Design review of the part built by this model. Coordinates are the model's own, in mm. A direction names the side the tool comes from. Give positions to 0.01 mm unless a question says otherwise; leave off trailing zeros. Loops run counter-clockwise (first coordinate to the right, second up) from the corner with the lowest first, then second, coordinate; pieces in that order, holes last. Notation, with made-up numbers: (30.5, -23.5) - (37.5, -23.5) arc R25 ccw to (37.5, 4.5) - close; hole circle Ø9 at (-39, 49). An arc over 180 degrees is marked (long way). Write each question's results on one line, items separated by ' | '.
from build123d import *

# Parameters (mm, degrees)
SKETCH1_R           = 3
BOSS_EXTRUDE1_DEPTH = 3.175


with BuildPart() as part:
    # Sketch1 → Boss-Extrude1 (new body)
    with BuildSketch(Plane.XY):
        with BuildLine():
            Line((25, 170), (175, 170))
            ThreePointArc((175, 170), (223.684930832, 189.383563894), (275, 200))
            Line((275, 200), (278.48892965, 170.203567833))
            ThreePointArc((278.48892965, 170.203567833), (228.984362684, 159.629140364), (182.323699215, 140))
            Line((182.323699215, 140), (17.676300785, 140))
            ThreePointArc((17.676300785, 140), (-27.163176857, 159.050053662), (-74.696057289, 169.732215313))
            add(Edge.make_bspline(
                [(-459.597813184, -125.74437106), (-458.167847661, -124.888859924), (-455.300989911, -123.160410804), (-449.693031194, -119.725805066), (-442.844497858, -115.430194443), (-434.897527213, -110.280573748), (-424.643042919, -103.410605598), (-412.446207366, -94.807407336), (-398.73286692, -84.425459971), (-385.875530014, -73.956655832), (-369.787206696, -59.850046206), (-355.152571956, -45.476802835), (-341.718077927, -30.784744771), (-332.160906415, -19.581186548), (-323.101555816, -8.241034683), (-311.630816912, 6.863649777), (-298.117522758, 25.605990916), (-282.395742384, 47.431562205), (-266.384320483, 68.25099024), (-249.34123977, 87.803395961), (-230.504956306, 105.928130356), (-212.601243201, 119.774018212), (-196.457396921, 130.048920131), (-183.303935629, 137.33205425), (-168.969219752, 144.162376514), (-153.317967868, 150.50005901), (-136.218766867, 156.296597686), (-120.658812709, 160.629761276), (-107.364076993, 163.767973943), (-96.958515184, 165.949209965), (-87.903435435, 167.618170459), (-80.445251901, 168.856738216), (-76.604810273, 169.448930821), (-74.696057289, 169.732215313)],
                knots=[0, 0, 0, 0, 0.007772041, 0.015544083, 0.031088165, 0.046632248, 0.06217633, 0.093264496, 0.124352661, 0.155440826, 0.186528991, 0.248705321, 0.279793487, 0.310881652, 0.341969817, 0.373057982, 0.435234312, 0.497410643, 0.559586973, 0.621763303, 0.683939634, 0.746115964, 0.777204129, 0.808292294, 0.83938046, 0.870468625, 0.90155679, 0.932644955, 0.948189038, 0.96373312, 0.979277203, 0.987049244, 0.994821285, 0.994821285, 0.994821285, 0.994821285], degree=3))
            Line((-459.597813184, -125.74437106), (-518.031074044, -125.74437106))
            Line((-518.031074044, -125.74437106), (-475, -100))
            add(Edge.make_bspline(
                [(-475, -100), (-419.540575809, -66.820070684), (-306.013905785, 34.036801702), (-257.635554762, 174.287094016), (-75, 200)],
                knots=[0, 0, 0, 0, 0.312223899, 1, 1, 1, 1], degree=3))
            ThreePointArc((-75, 200), (-23.684930832, 189.383563894), (25, 170))
        make_face()
        with Locations((-412.174499428, -75.74437106)):
            Circle(SKETCH1_R, mode=Mode.SUBTRACT)
        with Locations((-317.601811803, 24.25562894)):
            Circle(SKETCH1_R, mode=Mode.SUBTRACT)
        with Locations((-231.096695012, 124.25562894)):
            Circle(SKETCH1_R, mode=Mode.SUBTRACT)
        with Locations((-127.411512689, 174.25562894)):
            Circle(SKETCH1_R, mode=Mode.SUBTRACT)
        with Locations((100, 155)):
            Circle(SKETCH1_R, mode=Mode.SUBTRACT)
        with Locations((226.311251147, 174.505328628)):
            Circle(SKETCH1_R, mode=Mode.SUBTRACT)
        with Locations((-25.392583218, 174.221837866)):
            Circle(SKETCH1_R, mode=Mode.SUBTRACT)
    extrude(amount=BOSS_EXTRUDE1_DEPTH)


solid = part.part
(1) Take a section at B-B on z = 1.8. Count the separate pieces of the cut face and the enclosed holes in it, plus the area to 3 significant figures.
Answers below:
separate pieces: 1 | enclosed holes: 7 | area: 26,600 mm2
(2) Insertion check: P1, Ø1.6, axis at x = 132, z = 2, coming from the +Y side; P2, Ø3.5, axis at x = -25.39, y = 174.22, coming from the -Z side; P3, Ø1, axis at x = 47.5, z = 1, coming from the -Y side; P4, Ø1, axis at x = 189, z = 2, coming from the -Y side. Each pin has a flat end and moves straight along its axis. Give the tip position at first contact, or say it passes through.
Answers below:
P1: y = 170 | P2: through | P3: y = 140 | P4: y = 143.21
(3) Take a section at A-A on x = 45. Give the boundary of the cut face in (y, z) (3 decimals).
Answers below:
outline: (140, 0) - (170, 0) - (170, 3.175) - (140, 3.175) - close
(4) Wall thickness on line 1 along Y through (x, z) = (100, 1); line 2 along X through (y, z) = (170.5, 1.55); line 3 along Y through (x, z) = (151, 2.2): over which ranges is each line inside the solid? List them lowest first. Write a range as from..to.
Answers below:
line 1: 140..152, 158..170 | line 2: -183.17..24, 176..278.45 | line 3: 140..170
(5) Draft analysis for pull direction X (two halves, no side actions). For faces 4 (the flat face through (-496.817, -113.052, 1.565)), 5 (the flat face through (-177, 146, 3.175)), 6 (the cylindrical face through (-24.389, 189.594, 1.565)), state which applies: pulls with the +X half, pulls with the -X half, needs draft (parallel to the pull), parting line crosses it, or undercut.
Answers below:
face 4: pulls with the -X half | face 5: needs draft | face 6: undercut
(6) Tool access review of faces 1 (the cylindrical face through (-26.51, 158.84, 1.57)), 2 (the cylindrical face through (222.98, 189.17, 1.57)), 3 (the cylindrical face through (229.66, 159.84, 1.57)): name each direction out of +Z, -Z, +X, -X, +Y, -Y from which nothing blocks a thin tool from reaching the whole face with its end or side.
Answers below:
face 1: +Z, -Z, -Y | face 2: +Z, -Z, +Y | face 3: +Z, -Z, +X, -Y
